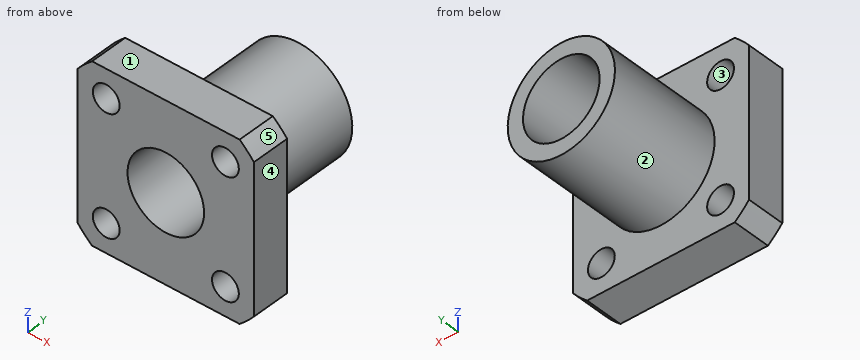
from build123d import *

# Parameters (mm, degrees)
SKETCH1_R           = 1.75
BOSS_EXTRUDE1_DEPTH = 5
SKETCH2_R           = 7
BOSS_EXTRUDE2_DEPTH = 15
SKETCH3_R           = 5
CUT_EXTRUDE1_DEPTH  = 26.777897509


with BuildPart() as part:
    # Sketch1 → Boss-Extrude1 (new body)
    with BuildSketch(Plane(origin=(0, 0, 0), x_dir=(1, 0, 0), z_dir=(0, 1, 0))):
        with BuildLine():
            Line((-9.630680142, -11.5), (9.630680142, -11.5))
            ThreePointArc((9.630680142, -11.5), (10.606601718, -10.606601718), (11.5, -9.630680142))
            Line((11.5, -9.630680142), (11.5, 9.630680142))
            ThreePointArc((11.5, 9.630680142), (10.606601718, 10.606601718), (9.630680142, 11.5))
            Line((9.630680142, 11.5), (-9.630680142, 11.5))
            ThreePointArc((-9.630680142, 11.5), (-10.606601718, 10.606601718), (-11.5, 9.630680142))
            Line((-11.5, 9.630680142), (-11.5, -9.630680142))
            ThreePointArc((-11.5, -9.630680142), (-10.606601718, -10.606601718), (-9.630680142, -11.5))
        make_face()
        with Locations(Location((-7.778174593, 7.778174593, 0), (0, 0, 270))):
            Circle(SKETCH1_R, mode=Mode.SUBTRACT)
        with Locations(Location((7.778174593, 7.778174593, 0), (0, 0, 270))):
            Circle(SKETCH1_R, mode=Mode.SUBTRACT)
        with Locations(Location((-7.778174593, -7.778174593, 0), (0, 0, 270))):
            Circle(SKETCH1_R, mode=Mode.SUBTRACT)
        with Locations(Location((7.778174593, -7.778174593, 0), (0, 0, 270))):
            Circle(SKETCH1_R, mode=Mode.SUBTRACT)
    extrude(amount=BOSS_EXTRUDE1_DEPTH)

    # Sketch2 → Boss-Extrude2 (add)
    with BuildSketch(Plane(origin=(0, 5, 0), x_dir=(1, 0, 0), z_dir=(0, 1, 0))):
        with Locations(Location((0, 0, 0), (0, 0, 270))):
            Circle(SKETCH2_R)
    extrude(amount=BOSS_EXTRUDE2_DEPTH)

    # Sketch3 → Cut-Extrude1 (cut, through all)
    with BuildSketch(Plane(origin=(0, 20, 0), x_dir=(1, 0, 0), z_dir=(0, 1, 0))):
        with Locations(Location((0, 0, 0), (0, 0, 270))):
            Circle(SKETCH3_R)
    extrude(amount=-CUT_EXTRUDE1_DEPTH, mode=Mode.SUBTRACT)


solid = part.part
Geometry check sheet. Reference: the model listing, model coordinates, mm. Face numbers are marked on the shaded views. A direction names the side the tool comes from. Round coordinates to 2 decimals unless told otherwise and drop trailing zeros. Write each loop counter-clockwise with the first axis right and the second up, starting at its lowest first coordinate (ties: lowest second). Pieces come first, ordered by that corner, then holes.
Item 1: Material ranges on line 1 along Z through (x, y) = (0.25, 1); line 2 along Y through (x, z) = (10.5, -2.75); line 3 along X through (y, z) = (6.5, -4), recorded low to high.
Determined:
line 1: z = -11.5 to -4.99, 4.99 to 11.5
line 2: y = 0 to 5
line 3: x = -5.74 to -3, 3 to 5.74
Item 2: Mould release check, pull along Z, two halves, no side actions. Record for the marked faces 3, 4 and 5: +Z half, -Z half, draft (parallel to the pull), parting line (faces both ways), or undercut.
Determined:
face 3: undercut
face 4: draft
face 5: +Z half
Item 3: Section check A-A (z = 0). Record the boundary of the cut face in (x, y).
Determined:
outline: (-11.5, 0) - (-5, 0) - (-5, 20) - (-7, 20) - (-7, 5) - (-11.5, 5) - close; (5, 0) - (11.5, 0) - (11.5, 5) - (7, 5) - (7, 20) - (5, 20) - close
Item 4: Access from +Z, -Z, +X, -X, +Y, -Y to the whole of each face (thin tool, end or side, straight path). Record for the marked faces 1 and 2.
Determined:
face 1: +Z, +X, -X, +Y, -Y
face 2: +Y
Item 5: Section check B-B (x = 0). Record the boundary of the cut face in (y, z).
Determined:
outline: (0, -11.5) - (5, -11.5) - (5, -7) - (20, -7) - (20, -5) - (0, -5) - close; (0, 5) - (20, 5) - (20, 7) - (5, 7) - (5, 11.5) - (0, 11.5) - close
Item 6: Go/stop test with flat-tipped pins: pin 1 Ø4 at (x, z) = (-7.78, 7.78) entering from +Y; pin 2 Ø8 at (y, z) = (17, 1.5) entering from -X; pin 3 Ø3 at (x, y) = (-0.5, 13.5) entering from +Z. Record where each tip stops, or that it passes through.
Determined:
pin 1: stops at y = 5
pin 2: stops at x = -7
pin 3: stops at z = 7
Item 7: Section check C-C (z = -7.75). Record the boundary of the cut face in (x, y), plus the area to 3 significant figures.
Determined:
outline: (-11.5, 0) - (-9.53, 0) - (-9.53, 5) - (-11.5, 5) - close; (-6.03, 0) - (6.03, 0) - (6.03, 5) - (-6.03, 5) - close; (9.53, 0) - (11.5, 0) - (11.5, 5) - (9.53, 5) - close
area: 80.0 mm2
Item 8: Section check D-D (y = 17.75). Record the boundary of the cut face in (x, z).
Determined:
outline: circle Ø14 at (0, 0); hole circle Ø10 at (0, 0)
